The listing builds one solid part. Answer for the finished solid, in the listing's coordinates (mm). Give positions to 0.01 mm unless a question says otherwise; leave off trailing zeros. Loops run counter-clockwise (first coordinate to the right, second up) from the corner with the lowest first, then second, coordinate; pieces in that order, holes last. Notation, with made-up numbers: M -16,34 L 21,34 A13 cw 21,39 Z; hole C 35.25,1 d10. An arc over 180 degrees is marked long. Return JSON: item names as keys, results as strings.
Autodesk Inventor part; units mm, degrees
ref_plane "YZ Plane" through (0, 0, 0) normal (1, 0, 0) x (0, 1, 0)
ref_plane "XZ Plane" through (0, 0, 0) normal (0, 1, 0) x (-1, 0, 0)
ref_plane "XY Plane" through (0, 0, 0) normal (0, 0, 1) x (1, 0, 0)
sketch "Sketch1" plane through (0, 0, 0) normal (0, 0, 1) x (1, 0, 0)
  circle A0 centre (0, 0) radius 12.7
  line L0 (-15.875, 15.875) -> (15.875, 15.875)
  line L1 (15.875, 15.875) -> (15.875, -15.875)
  line L2 (15.875, -15.875) -> (-15.875, -15.875)
  line L3 (-15.875, -15.875) -> (-15.875, 15.875)
  line L4 (-15.875, 15.875) -> (15.875, -15.875) construction
  line L5 (15.875, 15.875) -> (-15.875, -15.875) construction
  line L6 (-15.875, 0) -> (15.875, 0)
  point P0 (-12.7, 0)
  point P1 (12.7, 0)
  dimension "d0" = 25.4
  dimension "d1" = 31.75
  dimension "d2" = 31.75
extrude "Extrusion1" add sketch "Sketch1" along normal blind 50.8 contours A0 L6 L3 L0 L1
sketch "Sketch2" plane through (-15.875, 15.875, 0) normal (0, 1, 0) x (1, 0, 0)
  line L0 (31.75, 0) -> (0, 0) construction
  line L1 (0, 0) -> (0, -50.8) construction
  line L2 (31.75, -50.8) -> (0, -50.8) construction
  line L3 (31.75, 0) -> (31.75, -50.8) construction
  line L4 (15.875, -50.8) -> (15.875, 0)
  point P0 (15.875, -38.1)
  point P1 (15.875, -12.7)
  point P2 (15.875, -25.4)
  dimension "d7" = 25.4
  dimension "d8" = 25.4
hole "Hole1" at (0, 15.875, 38.1) at (0, 15.875, 12.7) direction (0, -1, 0) diameter 5.7912 end through all
fillet "Fillet1" radius 2 4 edges at (15.875, 0, 25.4) (12.7, 0, 25.4) (-15.875, 0, 25.4) (-12.7, 0, 25.4)
fillet "Fillet2" radius 2 10 edges at (-14.2101, 2.8831, 50.8) (0, 12.7, 50.8) (14.2101, 2.8831, 50.8) (15.875, 10.3649, 50.8) (-15.875, 10.3649, 50.8) (-14.2101, 2.8831, 0) (0, 12.7, 0) (14.2101, 2.8831, 0) (15.875, 10.3649, 0) (-15.875, 10.3649, 0)
equation "\"d0\" = tubeOD"
equation "\"d3\" = attachmentLength"
equation "\"tubeOD\" = 25.4"
equation "\"attachmentLength\" = 50.8"
properties part number "Pipe Adapter" material "ABS Plastic"
(1) Given pin 1 (3 mm diameter, centred on x = 9.5, y = 6.5, fed in from +Z); pin 2 (2 mm diameter, centred on x = 2, z = 30, fed in from -Y); pin 3 (6 mm diameter, centred on x = -0.5, z = 29, fed in from -Y), each flat-ended and moving along its own axis, determine where each tip first touches the part or whether it passes through.
Values follow:
{"pin 1": "z = 49.87", "pin 2": "y = 12.34", "pin 3": "y = 12.21"}
(2) Straight lines are drawn through the part: line 1 along Z through (x, y) = (0, 14.65); line 2 along Z through (x, y) = (0, 14.15); line 3 along X through (y, z) = (14.55, 12.7) (3 decimals). For each, find the intervals that lie inside material, in ascending order.
Values follow:
{"line 1": "0 to 9.8, 15.6 to 35.2, 41 to 50.8", "line 2": "0.08 to 9.8, 15.6 to 35.2, 41 to 50.72", "line 3": "-15.875 to -2.896, 2.896 to 15.875"}
(3) The part is cut by section A-A (x = 0). Determine the outline of the cut face in (y, z) (3 decimals), and give its area (3 significant figures).
Values follow:
{"outline": "M 12.7,2 A2 ccw 14.7,0 L 15.875,0 L 15.875,9.804 L 12.7,9.804 Z; M 12.7,15.596 L 15.875,15.596 L 15.875,35.204 L 12.7,35.204 Z; M 12.7,40.996 L 15.875,40.996 L 15.875,50.8 L 14.7,50.8 A2 ccw 12.7,48.8 Z", "area": "123 mm²"}
(4) Determine the mould class of faces 1 (the flat face through (0, 15.875, 25)), 2 (the flat face through (0, 15, 0)), 3 (the cylindrical face through (1.109, 14.095, 40.775)), 4 (the flat face through (0, 15, 50.8)) for opening direction Z: released by +Z, released by -Z, zero draft, split by the parting line, or undercut.
Values follow:
{"face 1": "zero draft", "face 2": "released by -Z", "face 3": "undercut", "face 4": "released by +Z"}
